from build123d import *

# Parameters (mm, degrees)
SKETCH1_W             = 68
SKETCH1_H             = 27
BOSS_EXTRUDE1_DEPTH   = 28
SKETCH2_R             = 6
CUT_EXTRUDE1_DEPTH    = 28
SKETCH3_R             = 8
CUT_EXTRUDE2_DEPTH    = 28
M8_TAPPED_HOLE1_D     = 6.8
M8_TAPPED_HOLE1_DEPTH = 15


with BuildPart() as part:
    # Sketch1 → Boss-Extrude1 (new body)
    with BuildSketch(Plane(origin=(0, 0, 0), x_dir=(1, 0, 0), z_dir=(0, 1, 0))):
        with Locations((34, 13.5)):
            Rectangle(SKETCH1_W, SKETCH1_H)
    extrude(amount=BOSS_EXTRUDE1_DEPTH)

    # Sketch2 → Cut-Extrude1 (cut)
    with BuildSketch(Plane.XY):
        with Locations((18, 14)):
            Circle(SKETCH2_R)
    extrude(amount=-CUT_EXTRUDE1_DEPTH, mode=Mode.SUBTRACT)

    # Sketch3 → Cut-Extrude2 (cut)
    with BuildSketch(Plane(origin=(0, 28, 0), x_dir=(1, 0, 0), z_dir=(0, 1, 0))):
        with Locations(Location((50, 13.5, 0), (0, 0, 270))):
            Circle(SKETCH3_R)
    extrude(amount=-CUT_EXTRUDE2_DEPTH, mode=Mode.SUBTRACT)

    # M8 Tapped Hole1
    with Locations(Plane(origin=(68, 0, 0), x_dir=(0, 0, -1), z_dir=(1, 0, 0))):
        with Locations((13.5, 14)):
            Hole(M8_TAPPED_HOLE1_D / 2, depth=M8_TAPPED_HOLE1_DEPTH)


solid = part.part
The listing builds one solid part. Answer for the finished solid, in the listing's coordinates (mm). Round coordinates to 2 decimals unless told otherwise and drop trailing zeros. Write each loop counter-clockwise with the first axis right and the second up, starting at its lowest first coordinate (ties: lowest second). Pieces come first, ordered by that corner, then holes. Notation, with made-up numbers: (-29, 87.25) - (23, 87.25) arc R22 cw to (23, 116.25) - close; hole circle Ø7 at (-23.75, 13). An arc over 180 degrees is marked (long way). Use one line per item in the form item = value. Start each with the question number.
Item 1: A flat-ended cylindrical pin translates along its axis: pin 1 Ø1 at (x, y) = (58, 17.5) entering from +Z. Find the tip coordinate at first contact, or state that the pin passes through.
Item 2: A cutting plane is placed at D-D (y = 24.25). Write down the section's boundary in (x, z).
Item 3: Find the intervals of material crossed by line 1 (Z direction, x = 65.5, y = 14); line 2 (Y direction, x = 18, z = -8.5); line 3 (Y direction, x = 61.5, z = -13.5), in increasing order. Write a range as [from, to].
Item 4: A cutting plane is placed at C-C (x = 18). Write down the section's boundary in (y, z).
Item 5: A cutting plane is placed at B-B (z = -13.5). Write down the section's boundary in (x, y), plus the area to 3 significant figures.
Item 6: A cutting plane is placed at A-A (y = 14). Write down the section's boundary in (x, z).
Item 7: Determine the mould class of faces 1 (the flat face through (34, 0, -14)), 2 (the flat face through (34, 28, -14)), 3 (the cylindrical face through (62.5, 14.1, -16.9)), 4 (the flat face through (68, 11, -16)) for opening direction Y: +Y half, -Y half, draft (parallel to the pull), parting line (faces both ways), or undercut.
The answers:
q1.pin_1 = 0
q2.outline = (0, -27) - (68, -27) - (68, 0) - (0, 0) - close; hole circle Ø16 at (50, -13.5)
q3.line_1 = [-27, -16.9], [-10.1, 0]
q3.line_2 = [0, 8], [20, 28]
q3.line_3 = [0, 10.6], [17.4, 28]
q4.outline = (0, -27) - (8, -27) - (8, 0) - (0, 0) - close; (20, -27) - (28, -27) - (28, 0) - (20, 0) - close
q5.outline = (0, 0) - (42, 0) - (42, 28) - (0, 28) - close; (58, 0) - (68, 0) - (68, 10.6) - (58, 10.6) - close; (58, 17.4) - (68, 17.4) - (68, 28) - (58, 28) - close; hole circle Ø12 at (18, 14)
q5.area = 1,270 mm^2
q6.outline = (0, -27) - (12, -27) - (12, 0) - (0, 0) - close; (24, -27) - (68, -27) - (68, -16.9) - (57.24, -16.9) arc R8 cw (long way) to (57.24, -10.1) - (68, -10.1) - (68, 0) - (24, 0) - close
q7.face_1 = -Y half
q7.face_2 = +Y half
q7.face_3 = undercut
q7.face_4 = draft
